Autodesk Inventor part; units mm, degrees
ref_plane "YZ Plane" through (0, 0, 0) normal (1, 0, 0) x (0, 1, 0)
ref_plane "XZ Plane" through (0, 0, 0) normal (0, 1, 0) x (-1, 0, 0)
ref_plane "XY Plane" through (0, 0, 0) normal (0, 0, 1) x (1, 0, 0)
sketch "Sketch1" plane through (0, 0, 0) normal (0, 0, 1) x (1, 0, 0)
  circle A0 centre (0, 0) radius 16
  circle A1 centre (0, 0) radius 9.5
  circle A2 centre (0, 9.5) radius 2.25
  circle A3 centre (-8.2272, 4.75) radius 2.25
  circle A4 centre (-8.2272, -4.75) radius 2.25
  circle A5 centre (0, -9.5) radius 2.25
  circle A6 centre (8.2272, -4.75) radius 2.25
  circle A7 centre (8.2272, 4.75) radius 2.25
  circle A8 centre (0, 0) radius 6
  dimension "d1" = 19
  dimension "d0" = 32
  dimension "d2" = 4.5
  dimension "d5" = 360
  dimension "d7" = 12
extrude "Extrusion1" add sketch "Sketch1" along normal blind 2 contours A0 | A1 A6 A5 A4 A3 A2 A7
properties part number "rotor_hub_retainer"
Could you check a few things on this model? Use its own coordinates, in mm. Round coordinates to 2 decimals unless told otherwise and drop trailing zeros. Loops run counter-clockwise (first coordinate to the right, second up) from the corner with the lowest first, then second, coordinate; pieces in that order, holes last. Notation, with made-up numbers: (-5, 40) -> (48, 40) arc R18 ccw to (48, 52) -> close; hole circle Ø2 at (33, -34). An arc over 180 degrees is marked (long way). Put each result on its own line as item: value.
Q1. I want a section at B-B on y = 1.5. Write out the boundary of the cut face in (x, z), and give its area (3 significant figures).
Checks:
outline: (-15.93, 0) -> (-5.81, 0) -> (-5.81, 2) -> (-15.93, 2) -> close; (5.81, 0) -> (15.93, 0) -> (15.93, 2) -> (5.81, 2) -> close
area: 40.5 mm2
Q2. Thinking about a two-plate mould opening in Y: for faces 1 (the flat face through (0, -7, 0)), 2 (the cylindrical face through (-6.081, 4.074, 0.986)), 3 (the cylindrical face through (-3.47, 15.62, 0.99)), which applies, pulls with the +Y half, pulls with the -Y half, needs draft (parallel to the pull), parting line crosses it, or undercut?
Checks:
face 1: needs draft
face 2: undercut
face 3: parting line crosses it
Q3. Please list where these lines run through material, in increasing order: line 1 (Y direction, x = 0, z = 1.5); line 2 (X direction, y = 4.75, z = 1.1); line 3 (Y direction, x = 7, z = 1.65). Write a range as from..to.
Checks:
line 1: -16..-11.75, -7.25..-6, 6..7.25, 11.75..16
line 2: -15.28..-10.48, -5.98..-3.67, 3.67..5.98, 10.48..15.28
line 3: -14.39..-6.64, -2.86..2.86, 6.64..14.39
Q4. I want a section at C-C on x = 5.5. Write out the boundary of the cut face in (y, z), and give its area (3 significant figures).
Checks:
outline: (-15.02, 0) -> (-2.4, 0) -> (-2.4, 2) -> (-15.02, 2) -> close; (2.4, 0) -> (15.02, 0) -> (15.02, 2) -> (2.4, 2) -> close
area: 50.5 mm2
Q5. For pin 1 Ø5 at (x, y) = (8.23, 4.75) entering from -Z; pin 2 Ø1 at (y, z) = (-4.5, 1) entering from +X, each with a flat end and sliding along its axis, tell me the tip position at first contact or that it passes through.
Checks:
pin 1: z = 0
pin 2: x = 15.49
Q6. I want a section at A-A on x = 0. Write out the boundary of the cut face in (y, z).
Checks:
outline: (-16, 0) -> (-11.75, 0) -> (-11.75, 2) -> (-16, 2) -> close; (-7.25, 0) -> (-6, 0) -> (-6, 2) -> (-7.25, 2) -> close; (6, 0) -> (7.25, 0) -> (7.25, 2) -> (6, 2) -> close; (11.75, 0) -> (16, 0) -> (16, 2) -> (11.75, 2) -> close
Q7. I want a section at D-D on z = 0.4. Write out the boundary of the cut face in (x, y), and give its area (3 significant figures).
Checks:
outline: circle Ø32 at (0, 0); hole circle Ø4.5 at (-8.23, -4.75); hole circle Ø4.5 at (-8.23, 4.75); hole circle Ø12 at (0, 0); hole circle Ø4.5 at (0, -9.5); hole circle Ø4.5 at (0, 9.5); hole circle Ø4.5 at (8.23, -4.75); hole circle Ø4.5 at (8.23, 4.75)
area: 596 mm2
